Can you work these out from the model? Positions are in its coordinate system, mm. Face numbers are marked on the shaded views. A direction names the side the tool comes from. Round coordinates to 2 decimals unless told otherwise and drop trailing zeros. Order: outer loops, then holes, each group sorted by start corner. A loop starts at its lowest first (then second) coordinate and runs counter-clockwise, first axis right, second up. Notation, with made-up numbers: M 86,89.25 L 129,89.25 A31 ccw 129,124.25 Z; hole C -33,-11.5 d5. An arc over 180 degrees is marked long. Answer as a JSON object with one key per item and string values. Group by question number.
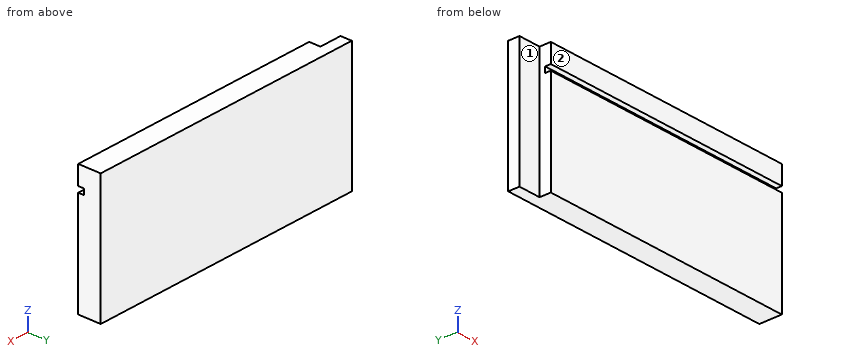
from build123d import *

# Parameters (mm, degrees)
F1_DEPTH = 150
F2_W     = 12
F2_H     = 6
F3_DEPTH = 68


with BuildPart() as f1:
    # F0 (on Right) → F1 (new body)
    with BuildSketch(Plane.YZ):
        Polygon((0, 55), (0, 0), (12, 0), (12, 68), (0, 68), (0, 58), (3, 58), (3, 55), align=None)
    extrude(amount=F1_DEPTH)

    # F2 (on Top) → F3 (cut)
    with BuildSketch(Plane.XY):
        with Locations((6, 3)):
            Rectangle(F2_W, F2_H)
    extrude(amount=F3_DEPTH, mode=Mode.SUBTRACT)


solid = f1.part
Item 1: On a 3-axis mill with a long thin cutter (end or side, diameter ignored), from which of +Z, -Z, +X, -X, +Y, -Y can I reach the whole of each face in a straight line? I mean the marked faces 1 and 2. Say none if no direction works.
Item 2: I need wall thicknesses on line 1 (Z direction, x = 16, y = 1.75); line 2 (X direction, y = 5.75, z = 29); line 3 (Y direction, x = 11, z = 24). Which ranges of each line are inside material? Lowest first, please.
Item 3: I'm going to push flat-ended pins straight in: pin 1 Ø2 at (y, z) = (3.5, 15.5) entering from -X; pin 2 Ø3.5 at (x, z) = (7.5, 19.5) entering from -Y; pin 3 Ø0.9 at (x, z) = (64.5, 56.5) entering from -Y. Where does each tip first touch, or does it pass through?
Item 4: Suppose I cut it at A-A, the plane z = 38. Write out the boundary of the cut face in (x, y).
Computed:
{
 "1": {"face 1": "+Z, -Z, -X, -Y", "face 2": "+Z, -Z, +X, -X, -Y"},
 "2": {"line 1": "z = 0 to 55, 58 to 68", "line 2": "x = 12 to 150", "line 3": "y = 6 to 12"},
 "3": {"pin 1": "stops at x = 12", "pin 2": "stops at y = 6", "pin 3": "stops at y = 3"},
 "4": {"outline": "M 0,6 L 12,6 L 12,0 L 150,0 L 150,12 L 0,12 Z"}
}
